Geometry: final body of the model. Coordinates: model frame, mm. Face numbers are marked on the shaded views. A direction names the side the tool comes from. Coordinates: 2 decimals unless noted, no trailing zeros. Order: outer loops, then holes, each group sorted by start corner. A loop starts at its lowest first (then second) coordinate and runs counter-clockwise, first axis right, second up. Notation, with made-up numbers: (-28, 54) -> (28, 54) arc R14 ccw to (28, 80) -> close; hole circle Ø2 at (-18, 26). An arc over 180 degrees is marked (long way). Answer in a Markdown table with one row per item. Add a question column.
1) Section query D-D on x = 4.5. Return the cut outline in (y, z), then the cut area to 3 significant figures.
2) Contact query for flat-ended pins moving along their axis: P1, Ø1.8, axis at y = 41, z = 0.5, coming from the +X side; P2, Ø0.9, axis at y = 40.5, z = 0, coming from the +X side; P3, Ø5.5, axis at x = -1.5, z = 0.5, coming from the -Y side. Output: stop coordinate, or through.
3) Section query A-A on z = 0. Count the separate pieces of the cut face and the enclosed holes in it, then the cut area to 3 significant figures.
4) Pull-direction query (Z, two-part tool) for the marked faces 1, 2 and 3; classes: +Z half, -Z half, draft (parallel to the pull), parting line (faces both ways), or undercut.
5) Ray query, line 1 (X direction, y = 20.5, z = -1.5); line 2 (X direction, y = 37, z = 0) (3 decimals); line 3 (Z direction, x = 6.1, y = 40.55). Return the intervals inside material, ascending. Write a range as from..to.
6) Set-up query: the marked faces 4, 5 and 6. Return all of +Z, -Z, +X, -X, +Y, -Y with unobstructed straight access to the full face (end or side cutting, diameter ignored); none if empty.
7) Section query B-B on y = 29.5. Return the cut outline in (x, z).
8) Section query C-C on z = -8. Return the cut outline in (x, y), then the cut area to 3 significant figures.
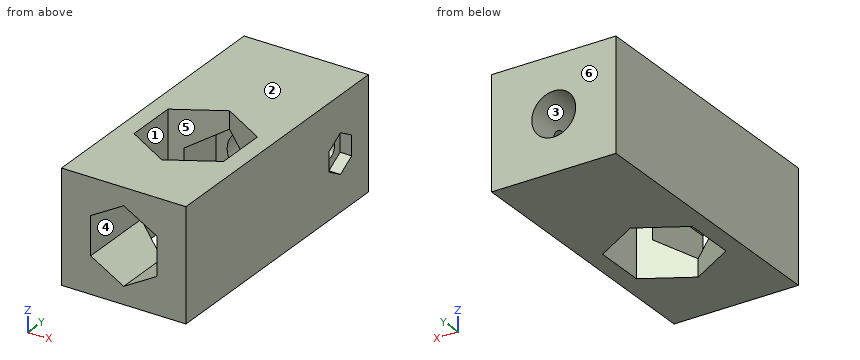
```python
from build123d import *

# Parameters (mm, degrees)
ESQUISSE1_W                  = 21.4
ESQUISSE1_H                  = 19.163586138
BOSS_EXTRU_1_DEPTH           = 47.9
ENL_V_MAT_EXTRU_1_DEPTH      = 32.9
ENL_V_MAT_EXTRU_2_REACH      = 49.9
ESQUISSE3_R                  = 3.775
ENL_V_MAT_EXTRU_3_DEPTH      = 1
ENL_V_MAT_EXTRU_3_DEPTH_BACK = 20.163586138
ESQUISSE5_R                  = 1.5
ENL_V_MAT_EXTRU_4_DEPTH      = 16
ENL_V_MAT_EXTRU_5_DEPTH      = 2


with BuildPart() as part:
    # Esquisse1 → Boss.-Extru.1 (new body)
    with BuildSketch(Plane(origin=(0, 0, 0), x_dir=(1, 0, 0), z_dir=(0, 1, 0))):
        Rectangle(ESQUISSE1_W, ESQUISSE1_H)
    extrude(amount=BOSS_EXTRU_1_DEPTH)

    # Esquisse2 → Enlèv. mat.-Extru.1 (cut)
    with BuildSketch(Plane(origin=(0, 0, 0), x_dir=(-1, 0, 0), z_dir=(0, -1, 0))):
        Polygon((5.7, -3.290896534), (0, -6.581793069), (-5.7, -3.290896534), (-5.7, 3.290896534), (0, 6.581793069), (5.7, 3.290896534), align=None)
    extrude(amount=-ENL_V_MAT_EXTRU_1_DEPTH, mode=Mode.SUBTRACT)

    # Esquisse3 → Enlèv. mat.-Extru.2 (cut, up to next)
    with BuildSketch(Plane(origin=(0, 47.9, 0), x_dir=(1, 0, 0), z_dir=(0, 1, 0)), mode=Mode.PRIVATE) as enl_v_mat_extru_2_sk1:
        with Locations(Location((0, 0, 0), (0, 0, 270))):  # turned: the seam where the file's is
            Circle(ESQUISSE3_R)
    enl_v_mat_extru_2_tool1 = extrude(enl_v_mat_extru_2_sk1.sketch, amount=-ENL_V_MAT_EXTRU_2_REACH, mode=Mode.PRIVATE) & part.part
    add(enl_v_mat_extru_2_tool1.solids().sort_by_distance((0, 47.9, 0))[0], mode=Mode.SUBTRACT)

    # Esquisse4 → Enlèv. mat.-Extru.3 (cut, two sides)
    with BuildSketch(Plane.XY.offset(9.581793069)) as enl_v_mat_extru_3_sk:
        Polygon((0, 27.782388291), (-7.7, 23.336791218), (-7.7, 14.445597073), (0, 10), (7.7, 14.445597073), (7.7, 23.336791218), align=None)
    extrude(amount=ENL_V_MAT_EXTRU_3_DEPTH, mode=Mode.SUBTRACT)
    extrude(enl_v_mat_extru_3_sk.sketch, amount=-ENL_V_MAT_EXTRU_3_DEPTH_BACK, mode=Mode.SUBTRACT)

    # Esquisse5 → Enlèv. mat.-Extru.4 (cut)
    with BuildSketch(Plane(origin=(10.7, 0, 0), x_dir=(0, 0, -1), z_dir=(1, 0, 0))):
        with Locations((0, 40.55)):
            Circle(ESQUISSE5_R)
    extrude(amount=-ENL_V_MAT_EXTRU_4_DEPTH, mode=Mode.SUBTRACT)

    # Esquisse6 → Enlèv. mat.-Extru.5 (cut)
    with BuildSketch(Plane(origin=(10.7, 0, 0), x_dir=(0, 0, -1), z_dir=(1, 0, 0))):
        Polygon((1.703183294, 43.5), (-1.703183294, 43.5), (-3.406366588, 40.55), (-1.703183294, 37.6), (1.703183294, 37.6), (3.406366588, 40.55), align=None)
    extrude(amount=-ENL_V_MAT_EXTRU_5_DEPTH, mode=Mode.SUBTRACT)


solid = part.part
```
Result:
| question | item | result |
|---|---|---|
| 1 | outline | (0, -9.58) -> (12.6, -9.58) -> (12.6, -3.98) -> (0, -3.98) -> close; (0, 3.98) -> (12.6, 3.98) -> (12.6, 9.58) -> (0, 9.58) -> close; (25.18, -9.58) -> (47.9, -9.58) -> (47.9, 9.58) -> (25.18, 9.58) -> (25.18, 3.98) -> (32.9, 3.98) -> (32.9, -3.98) -> (25.18, -3.98) -> close; hole circle Ø3 at (40.55, 0) |
| 1 | area | 508 mm2 |
| 2 | P1 | x = 8.7 |
| 2 | P2 | x = -5.3 |
| 2 | P3 | y = 32.9 |
| 3 | separate pieces | 3 |
| 3 | enclosed holes | 0 |
| 3 | area | 465 mm2 |
| 4 | face 1 | draft |
| 4 | face 2 | +Z half |
| 4 | face 3 | undercut |
| 5 | line 1 | -10.7..-7.7, 7.7..10.7 |
| 5 | line 2 | -10.7..-3.775, 3.775..10.7 |
| 5 | line 3 | -9.58..-1.5, 1.5..9.58 |
| 6 | face 4 | -Y |
| 6 | face 5 | +Z, -Z |
| 6 | face 6 | +Z, -Z, +X, -X, +Y |
| 7 | outline | (-10.7, -9.58) -> (10.7, -9.58) -> (10.7, 9.58) -> (-10.7, 9.58) -> close; hole (-5.7, -3.29) -> (0, -6.58) -> (5.7, -3.29) -> (5.7, 3.29) -> (0, 6.58) -> (-5.7, 3.29) -> close |
| 8 | outline | (-10.7, 0) -> (10.7, 0) -> (10.7, 47.9) -> (-10.7, 47.9) -> close; hole (-7.7, 14.45) -> (0, 10) -> (7.7, 14.45) -> (7.7, 23.34) -> (0, 27.78) -> (-7.7, 23.34) -> close |
| 8 | area | 820 mm2 |
